Input: part model. Units: mm. Frame: model coordinates. Coordinates: 2 decimals unless noted, no trailing zeros. Write each loop counter-clockwise with the first axis right and the second up, starting at its lowest first coordinate (ties: lowest second). Pieces come first, ordered by that corner, then holes.
1) Section query A-A (y = 9.5). Output: boundary loops of the cut face in (x, z), then the cut area to 3 significant figures.
2) Line query: L1, parallel to Y at x = -24, z = 0.4; L2, parallel to X at y = 3, z = 1.85; L3, parallel to X at y = -23.5, z = 1.65. Output: solid intervals per line, ascending.
3) Pin query (flat end, axial travel): pin 1 Ø3 at (x, y) = (16.28, 17.45) entering from +Z. Return the tip coordinate at first contact, or that it passes through.
4) Section query B-B (z = 0.6). State how many separate pieces and enclosed holes the cut face has, then the cut area to 3 significant figures.
5) Draft query along X for faces 1 (the cylindrical face through (-6.85, -40.11, 0.99)), 2 (the cylindrical face through (96.06, -52.36, 1.01)), 3 (the cylindrical face through (-52.19, 16.52, 0.99)). Return one class per face: pulls with the +X half, pulls with the -X half, needs draft (parallel to the pull), parting line crosses it, or undercut.
from build123d import *

# Parameters (mm, degrees)
F0_R     = 6
F0_R_2   = 2
F0_R_3   = 9.5
F1_DEPTH = 2
F2_R     = 5


# Not quite as in the source:
# - ends of sketch curves that miss each other by under 0.0002 mm in the source are joined


with BuildPart() as f1:
    # F0 (on Top) → F1 (new body)
    with BuildSketch(Plane.XY):
        Polygon((-23.8795465221, 51.1389637595), (-63.8795465221, 51.1389552037), (-63.8795465221, -53.8610447963), (-23.8795465221, -53.8610362327), (-23.3432798734, -53.8610447963), (16.1204534779, -53.861027669), (16.6553473944, -53.8610447963), (56.8043348949, -53.8610189589), (57.3406015435, -53.8610101337), (97.4896168807, -53.8610102485), (97.4896168807, 51.1389898663), (57.4896168808, 51.1389811639), (56.8043348949, 51.1389898663), (16.8043627316, 51.1389724616), (16.1204534779, 51.1389552037), (-23.1942645362, 51.138963906), align=None)
        with Locations((-48.9755360277, -32.7236170491)):
            Circle(F0_R, mode=Mode.SUBTRACT)
        with BuildLine():
            ThreePointArc((-40.2649926355, -27.7236170491), (-46.7743509608, -25.4265127742), (-50.3515408057, -19.5229421029))
            Line((-50.3515408057, -19.5229421029), (-27.0517710596, -19.6233615279))
            Line((-27.0517710596, -19.6233615279), (-27.0517710596, -45.6233615279))
            Line((-27.0517710596, -45.6233615279), (-50.3515408057, -45.9242919952))
            ThreePointArc((-50.3515408057, -45.9242919952), (-46.7743509608, -40.020721324), (-40.2649926355, -37.7236170491))
            Line((-40.2649926355, -37.7236170491), (-40.2649926355, -27.7236170491))
        make_face(mode=Mode.SUBTRACT)
        with Locations((-8.9769087599, -32.7076169273)):
            Circle(F0_R, mode=Mode.SUBTRACT)
        with BuildLine():
            ThreePointArc((-0.2663653677, -27.7076169273), (-6.7763425011, -25.3676442405), (-10.2489610341, -19.3846520981))
            Line((-10.2489610341, -19.3846520981), (6.5472276519, -22.2309003302))
            Line((6.5472276519, -22.2309003302), (6.5472276519, -45.2309003302))
            Line((6.5472276519, -45.2309003302), (-10.2489610341, -46.0305817564))
            ThreePointArc((-10.2489610341, -46.0305817564), (-6.7763425011, -40.047589614), (-0.2663653677, -37.7076169273))
            Line((-0.2663653677, -37.7076169273), (-0.2663653677, -27.7076169273))
        make_face(mode=Mode.SUBTRACT)
        with Locations((-54.0347284068, -19.0128381198)):
            Circle(F0_R_2, mode=Mode.SUBTRACT)
        with Locations((-23.7243646373, -19.0128381198)):
            Circle(F0_R_2, mode=Mode.SUBTRACT)
        with Locations((-14.0347284068, -19.1747317856)):
            Circle(F0_R_2, mode=Mode.SUBTRACT)
        with Locations((16.2756353627, -19.1747317856)):
            Circle(F0_R_2, mode=Mode.SUBTRACT)
        with Locations((31.7083453892, -32.7075822646)):
            Circle(F0_R, mode=Mode.SUBTRACT)
        with BuildLine():
            ThreePointArc((40.4188887821, -27.7075822646), (33.9089116483, -25.3676095781), (30.436293115, -19.3846174354))
            Line((30.436293115, -19.3846174354), (47.2324818011, -22.2308656676))
            Line((47.2324818011, -22.2308656676), (47.2324818011, -45.2308656676))
            Line((47.2324818011, -45.2308656676), (30.436293115, -46.0305470938))
            ThreePointArc((30.436293115, -46.0305470938), (33.9089116483, -40.0475549511), (40.4188887821, -37.7075822646))
            Line((40.4188887821, -37.7075822646), (40.4188887821, -27.7075822646))
        make_face(mode=Mode.SUBTRACT)
        with Locations((72.393430969, -32.7070186107)):
            Circle(F0_R, mode=Mode.SUBTRACT)
        with BuildLine():
            ThreePointArc((81.1039743612, -27.7070186107), (74.5943131753, -25.3674773264), (71.1213786947, -19.3851810893))
            Line((71.1213786947, -19.3851810893), (87.9175673808, -22.2314293214))
            Line((87.9175673808, -22.2314293214), (87.9175673808, -45.2314293214))
            Line((87.9175673808, -45.2314293214), (71.1213786947, -46.0288561321))
            ThreePointArc((71.1213786947, -46.0288561321), (74.5943131753, -40.046559895), (81.1039743612, -37.7070186107))
            Line((81.1039743612, -37.7070186107), (81.1039743612, -27.7070186107))
        make_face(mode=Mode.SUBTRACT)
        with Locations((26.6491530101, -19.1746971229)):
            Circle(F0_R_2, mode=Mode.SUBTRACT)
        with Locations((67.334434996, -19.1746971229)):
            Circle(F0_R_2, mode=Mode.SUBTRACT)
        with Locations((-54.0347284068, -0.8610447963)):
            Circle(F0_R_2, mode=Mode.SUBTRACT)
        with Locations((-41.5101771743, 3.8599752962)):
            Circle(F0_R_3, mode=Mode.SUBTRACT)
        with Locations((-23.7243646373, -0.8610447963)):
            Circle(F0_R_2, mode=Mode.SUBTRACT)
        with Locations((-54.0347284068, 17.2907485271)):
            Circle(F0_R_2, mode=Mode.SUBTRACT)
        with Locations((-23.7243646373, 17.2907485271)):
            Circle(F0_R_2, mode=Mode.SUBTRACT)
        with Locations((-14.0347284068, -0.8610447963)):
            Circle(F0_R_2, mode=Mode.SUBTRACT)
        with Locations((-1.5101771743, 3.8599752962)):
            Circle(F0_R_3, mode=Mode.SUBTRACT)
        with Locations((16.2756353627, -0.8610447963)):
            Circle(F0_R_2, mode=Mode.SUBTRACT)
        with Locations((-14.0347284068, 17.4526421929)):
            Circle(F0_R_2, mode=Mode.SUBTRACT)
        with Locations((16.2756353627, 17.4526421929)):
            Circle(F0_R_2, mode=Mode.SUBTRACT)
        with Locations((-48.9755360277, 31.0015274564)):
            Circle(F0_R, mode=Mode.SUBTRACT)
        with BuildLine():
            ThreePointArc((-40.2649926355, 36.0015274564), (-46.7743509608, 38.2986317313), (-50.3515408057, 44.2022024026))
            Line((-50.3515408057, 44.2022024026), (-27.0517710596, 43.9012719352))
            Line((-27.0517710596, 43.9012719352), (-27.0517710596, 17.9012719352))
            Line((-27.0517710596, 17.9012719352), (-31.7607614923, 17.8809767084))
            Line((-31.7607614923, 17.8809767084), (-31.7607756326, 17.7187155905))
            ThreePointArc((-31.7607756326, 17.7187155905), (-31.7603267926, 17.6887571457), (-31.7601771743, 17.6587957124))
            ThreePointArc((-31.7601771743, 17.6587957124), (-34.7601771743, 14.6587957124), (-37.7601771743, 17.6587957124))
            Line((-37.7601771743, 17.6587957124), (-37.7601771743, 17.8551198918))
            Line((-37.7601771743, 17.8551198918), (-50.3515408057, 17.8008525103))
            ThreePointArc((-50.3515408057, 17.8008525103), (-46.7743509608, 23.7044231815), (-40.2649926355, 26.0015274564))
            Line((-40.2649926355, 26.0015274564), (-40.2649926355, 36.0015274564))
        make_face(mode=Mode.SUBTRACT)
        with Locations((-8.9769087599, 30.9855273346)):
            Circle(F0_R, mode=Mode.SUBTRACT)
        with BuildLine():
            ThreePointArc((-0.2663653677, 35.9855273346), (-6.7763425011, 38.3255000213), (-10.2489610341, 44.3084921637))
            Line((-10.2489610341, 44.3084921637), (6.5472276519, 43.5088107375))
            Line((6.5472276519, 43.5088107375), (6.5472276519, 27.1076551873))
            ThreePointArc((6.5472276519, 27.1076551873), (7.7807259121, 26.0009361033), (8.2384500935, 24.4081920365))
            Line((8.2384500935, 24.4081920365), (8.2378516352, 17.5408218029))
            ThreePointArc((8.2378516352, 17.5408218029), (8.2383004752, 17.5108633581), (8.2384500935, 17.4809019247))
            ThreePointArc((8.2384500935, 17.4809019247), (5.2384500935, 14.4809019247), (2.2384500935, 17.4809019247))
            Line((2.2384500935, 17.4809019247), (2.2384500935, 19.7786539896))
            Line((2.2384500935, 19.7786539896), (-10.2489610341, 17.6625625054))
            ThreePointArc((-10.2489610341, 17.6625625054), (-6.7763425011, 23.6455546479), (-0.2663653677, 25.9855273346))
            Line((-0.2663653677, 25.9855273346), (-0.2663653677, 35.9855273346))
        make_face(mode=Mode.SUBTRACT)
        with Locations((26.6491530101, -0.8610101337)):
            Circle(F0_R_2, mode=Mode.SUBTRACT)
        with Locations((39.1737042426, 3.8600099589)):
            Circle(F0_R_3, mode=Mode.SUBTRACT)
        with Locations((26.6491530101, 17.4526768556)):
            Circle(F0_R_2, mode=Mode.SUBTRACT)
        with Locations((67.334434996, -0.8610101337)):
            Circle(F0_R_2, mode=Mode.SUBTRACT)
        with Locations((79.8589862285, 3.8600099589)):
            Circle(F0_R_3, mode=Mode.SUBTRACT)
        with Locations((67.334434996, 17.4526768556)):
            Circle(F0_R_2, mode=Mode.SUBTRACT)
        with Locations((31.7083453892, 30.9855619972)):
            Circle(F0_R, mode=Mode.SUBTRACT)
        with BuildLine():
            ThreePointArc((40.4188887821, 35.9855619972), (33.9089116483, 38.3255346838), (30.436293115, 44.3085268264))
            Line((30.436293115, 44.3085268264), (47.2324818011, 43.5088454002))
            Line((47.2324818011, 43.5088454002), (47.2324818011, 27.10768985))
            ThreePointArc((47.2324818011, 27.10768985), (48.4659800612, 26.000970766), (48.9237042426, 24.4082266992))
            Line((48.9237042426, 24.4082266992), (48.9231057843, 17.5408564655))
            ThreePointArc((48.9231057843, 17.5408564655), (48.9235546243, 17.5108980207), (48.9237042426, 17.4809365874))
            ThreePointArc((48.9237042426, 17.4809365874), (45.9237042426, 14.4809365874), (42.9237042426, 17.4809365874))
            Line((42.9237042426, 17.4809365874), (42.9237042426, 19.7786886523))
            Line((42.9237042426, 19.7786886523), (30.436293115, 17.6625971681))
            ThreePointArc((30.436293115, 17.6625971681), (33.9089116483, 23.6455893107), (40.4188887821, 25.9855619972))
            Line((40.4188887821, 25.9855619972), (40.4188887821, 35.9855619972))
        make_face(mode=Mode.SUBTRACT)
        with Locations((72.393430969, 30.9849983434)):
            Circle(F0_R, mode=Mode.SUBTRACT)
        with BuildLine():
            ThreePointArc((81.1039743612, 35.9849983434), (74.5943131753, 38.3245396276), (71.1213786947, 44.3068358648))
            Line((71.1213786947, 44.3068358648), (87.9175673808, 43.5094090541))
            Line((87.9175673808, 43.5094090541), (87.9175673808, 27.1071261961))
            ThreePointArc((87.9175673808, 27.1071261961), (89.151065641, 26.0004071121), (89.6087898224, 24.4076630453))
            Line((89.6087898224, 24.4076630453), (89.6081913641, 17.5402928116))
            ThreePointArc((89.6081913641, 17.5402928116), (89.6086402041, 17.5103343668), (89.6087898224, 17.4803729335))
            ThreePointArc((89.6087898224, 17.4803729335), (86.6087898224, 14.4803729335), (83.6087898224, 17.4803729335))
            Line((83.6087898224, 17.4803729335), (83.6087898224, 19.7792523062))
            Line((83.6087898224, 19.7792523062), (71.1213786947, 17.663160822))
            ThreePointArc((71.1213786947, 17.663160822), (74.5943131753, 23.6454570591), (81.1039743612, 25.9849983434))
            Line((81.1039743612, 25.9849983434), (81.1039743612, 35.9849983434))
        make_face(mode=Mode.SUBTRACT)
    extrude(amount=F1_DEPTH)

    # F2
    f2_edges = [f1.edges().sort_by_distance(p)[0] for p in [
        (-63.879547, 51.138955, 1),
        (97.489617, 51.13899, 1),
        (-63.879547, -53.861045, 1),
        (97.489617, -53.86101, 1),
    ]]
    fillet(f2_edges, radius=F2_R)


solid = f1.part
Answer:
1. outline: (-63.88, 0) - (-49.15, 0) - (-49.15, 2) - (-63.88, 2) - close; (-33.87, 0) - (-9.15, 0) - (-9.15, 2) - (-33.87, 2) - close; (6.13, 0) - (31.53, 0) - (31.53, 2) - (6.13, 2) - close; (46.82, 0) - (72.21, 0) - (72.21, 2) - (46.82, 2) - close; (87.5, 0) - (97.49, 0) - (97.49, 2) - (87.5, 2) - close
1. area: 200 mm2
2. L1: y = -53.86 to -20.99, -17.03 to -2.84, 1.12 to 15.31, 19.27 to 51.14
2. L2: x = -63.88 to -50.97, -32.05 to -10.97, 7.95 to 29.71, 48.63 to 70.4, 89.32 to 97.49
2. L3: x = -63.88 to -48.6, -27.05 to -8.51, 6.55 to 32.17, 47.23 to 72.86, 87.92 to 97.49
3. pin 1: passes through
4. separate pieces: 1
4. enclosed holes: 38
4. area: 11,900 mm2
5. face 1: undercut
5. face 2: pulls with the +X half
5. face 3: undercut
